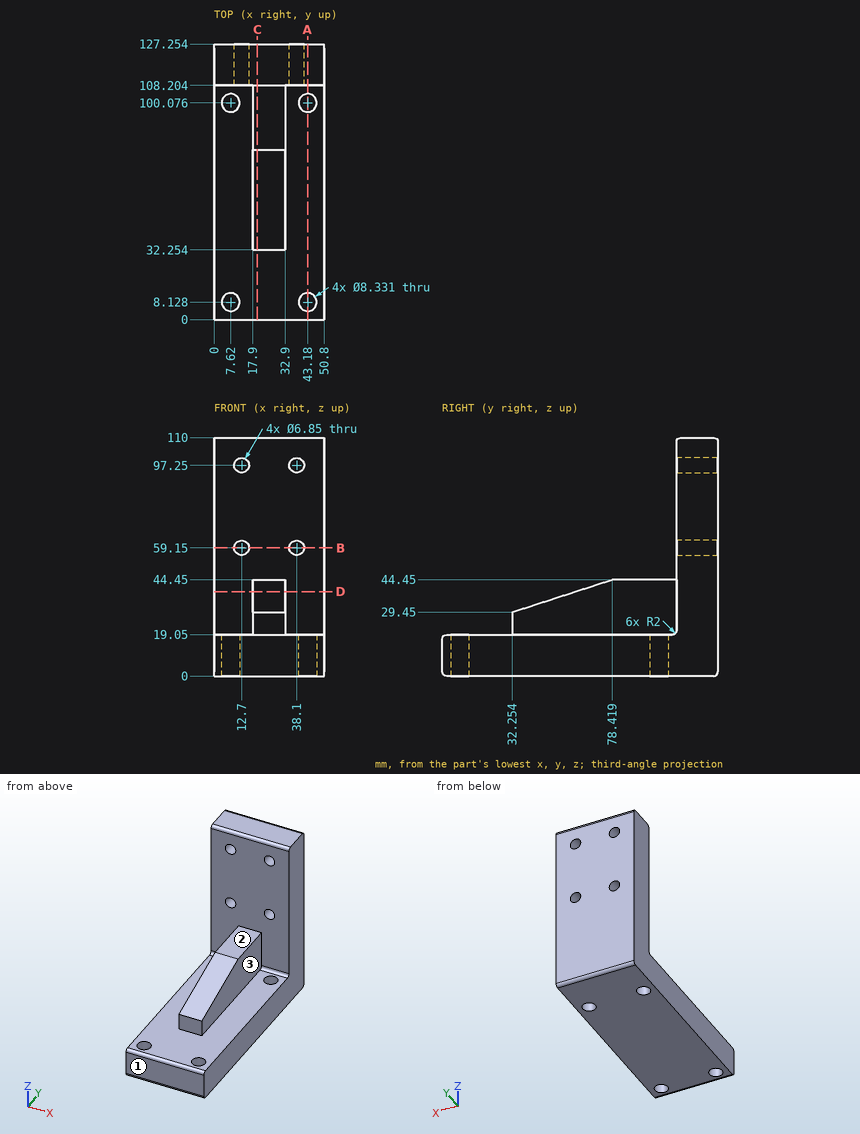
Part print with two shaded views. Sizes in mm from the minimum x, y, z corner. A direction names the side the tool comes from. Coordinates: 2 decimals unless noted, no trailing zeros. Write each loop counter-clockwise with the first axis right and the second up, starting at its lowest first coordinate (ties: lowest second). Pieces come first, ordered by that corner, then holes. Notation, with made-up numbers: (40, -26) - (55, -26) arc R11 ccw to (55, -14) - close; hole circle Ø6 at (-18.75, 1.25). An arc over 180 degrees is marked (long way). Put each result on its own line as item: value.
1. Band-saw the part on B-B (z = 59.15). Write the cut outline in (x, y) (1 decimal), then the cut area to 3 significant figures.
Final values:
outline: (0, 108.2) - (9.3, 108.2) - (9.3, 127.3) - (0, 127.3) - close; (16.1, 108.2) - (34.7, 108.2) - (34.7, 127.3) - (16.1, 127.3) - close; (41.5, 108.2) - (50.8, 108.2) - (50.8, 127.3) - (41.5, 127.3) - close
area: 707 mm²
2. Band-saw the part on A-A (x = 43.18). Write the cut outline in (y, z).
Final values:
outline: (0, 2) arc R2 ccw to (2, 0) - (3.96, 0) - (3.96, 19.05) - (2, 19.05) arc R2 ccw to (0, 17.05) - close; (12.29, 0) - (95.91, 0) - (95.91, 19.05) - (12.29, 19.05) - close; (104.24, 0) - (125.25, 0) arc R2 ccw to (127.25, 2) - (127.25, 108) arc R2 ccw to (125.25, 110) - (110.2, 110) arc R2 ccw to (108.2, 108) - (108.2, 21.05) arc R2 cw to (106.2, 19.05) - (104.24, 19.05) - close
3. 3-axis set-ups, long thin cutter, end or side, ignore diameter. For the marked faces 1, 2 and 3: which of +Z, -Z, +X, -X, +Y, -Y reach the whole face in a straight line?
Final values:
face 1: +Z, -Z, +X, -X, -Y
face 2: +Z, +X, -X, -Y
face 3: +Z, +X, -Y
4. Probe line 1 along X through (y, z) = (118.5, 97.25) (1 decimal); line 2 along Y through (x, z) = (43, 4); line 3 along Z through (x, y) = (26, 23). List the from-to ranges inside material, lowest first. Write a range as [from, to].
Final values:
line 1: x = [0, 9.3], [16.1, 34.7], [41.5, 50.8]
line 2: y = [0, 3.97], [12.29, 95.91], [104.24, 127.25]
line 3: z = [0, 19.05]
5. Band-saw the part on D-D (z = 39). Write the cut outline in (x, y), then the cut area to 3 significant figures.
Final values:
outline: (0, 108.2) - (17.9, 108.2) - (17.9, 61.65) - (32.9, 61.65) - (32.9, 108.2) - (50.8, 108.2) - (50.8, 127.25) - (0, 127.25) - close
area: 1,670 mm²
6. Flat gauge pins, fed straight in: pin 1 Ø8 at (y, z) = (38, 31) entering from -X; pin 2 Ø8 at (x, z) = (12.7, 59.15) entering from -Y; pin 3 Ø4.5 at (x, y) = (22, 89) entering from +Z; pin 4 Ø6 at (x, z) = (12.7, 97.25) entering from -Y. Where does each tip first touch, or does it go through?
Final values:
pin 1: stops at x = 17.9
pin 2: stops at y = 108.2
pin 3: stops at z = 44.45
pin 4: passes through
7. Band-saw the part on C-C (x = 20). Write the cut outline in (y, z).
Final values:
outline: (0, 2) arc R2 ccw to (2, 0) - (125.25, 0) arc R2 ccw to (127.25, 2) - (127.25, 108) arc R2 ccw to (125.25, 110) - (110.2, 110) arc R2 ccw to (108.2, 108) - (108.2, 44.45) - (78.42, 44.45) - (32.25, 29.45) - (32.25, 19.05) - (2, 19.05) arc R2 ccw to (0, 17.05) - close
